Read the model definition and answer for the solid it produces. Units are mm, in the model's axes. Coordinates: 2 decimals unless noted, no trailing zeros. Write each loop counter-clockwise with the first axis right and the second up, starting at its lowest first coordinate (ties: lowest second). Pieces come first, ordered by that corner, then holes. Notation, with made-up numbers: (69.25, 49.25) -> (81.25, 49.25) arc R15 cw to (81.25, 56.25) -> close; hole circle Ø8 at (-0.75, 66.5). An arc over 180 degrees is marked (long way). Answer in a Markdown table with one row per item. Add a question column.
Item 1: For a pull along Z with two mould halves and no side action, classify faces 1 (the face through (-5, 4, -4)), 2 (the face through (-4.346, 1.972, -0.834)), 3 (the face through (5.854, 3.865, -14.543)) as +Z half, -Z half, draft (parallel to the pull), parting line (faces both ways), or undercut.
Item 2: Section A-A on z = -1.5 is taken. Write down the section's boundary in (x, y).
Item 3: Straight lines are drawn through the part: line 1 (X direction, y = 1.35, z = -0.5); line 2 (Z direction, x = 3, y = 3.55); line 3 (Z direction, x = 5.5, y = 2.65). For each, find the intervals that lie inside material, in ascending order. Write a range as from..to.
Item 4: Section B-B on y = 2.25 is taken. Write down the section's boundary in (x, z), then the cut area to 3 significant figures.
```python
from build123d import *

# Parameters (mm, degrees)
SKETCH1_W                      = 25
SKETCH1_H                      = 25
BOSS_EXTRUDE1_DEPTH            = 4
FILLET1_R                      = 4
F_1_7_1_7_DIAMETER_HOLE1_D     = 1.7
F_1_7_1_7_DIAMETER_HOLE1_DEPTH = 8.5
CHAMFER1_SIZE                  = 0.5


with BuildPart() as part:
    # Sketch1 → Boss-Extrude1 (new body)
    with BuildSketch(Plane(origin=(0, 0, 0), x_dir=(1, 0, 0), z_dir=(0, 1, 0))):
        with Locations((-5.188287333, 3.444371681)):
            Rectangle(SKETCH1_W, SKETCH1_H)
    extrude(amount=BOSS_EXTRUDE1_DEPTH)

    # Fillet1
    fillet1_edges = [part.edges().sort_by_distance(p)[0] for p in [
        (-17.688287333, 2, -15.944371681),
        (7.311712667, 2, -15.944371681),
        (7.311712667, 2, 9.055628319),
        (-17.688287333, 2, 9.055628319),
    ]]
    fillet(fillet1_edges, radius=FILLET1_R)

    # Ø1.7 (1.7) Diameter Hole1
    with Locations(Plane(origin=(-5.188287333, 4, -0.944371681), x_dir=(0, 0, 1), z_dir=(0, 1, 0))):
        with Locations((0, 0)):
            Hole(F_1_7_1_7_DIAMETER_HOLE1_D / 2, depth=F_1_7_1_7_DIAMETER_HOLE1_DEPTH)

    # Chamfer1
    chamfer1_edges = [part.edges().sort_by_distance(p)[0] for p in [
        (-17.688287333, 0, -3.444371681),
        (-17.688287333, 4, -3.444371681),
        (-5.188287333, 0, -15.944371681),
        (7.311712667, 0, -3.444371681),
        (-5.188287333, 0, 9.055628319),
        (-16.516714458, 0, 7.884055444),
        (6.140139792, 0, 7.884055444),
        (6.140139792, 0, -14.772798805),
        (-16.516714458, 0, -14.772798805),
        (-5.188287333, 4, -15.944371681),
        (-5.188287333, 4, 9.055628319),
        (7.311712667, 4, -3.444371681),
        (-16.516714458, 4, 7.884055444),
        (6.140139792, 4, 7.884055444),
        (6.140139792, 4, -14.772798805),
        (-16.516714458, 4, -14.772798805),
    ]]
    chamfer(chamfer1_edges, length=CHAMFER1_SIZE)


solid = part.part
```
Results below:
| question | item | result |
|---|---|---|
| 1 | face 1 | draft |
| 1 | face 2 | undercut |
| 1 | face 3 | -Z half |
| 2 | outline | (-17.69, 0.5) -> (-17.19, 0) -> (-5.83, 0) -> (-5.83, 4) -> (-17.19, 4) -> (-17.69, 3.5) -> close; (-4.55, 0) -> (6.81, 0) -> (7.31, 0.5) -> (7.31, 3.5) -> (6.81, 4) -> (-4.55, 4) -> close |
| 3 | line 1 | x = -17.69..-5.91, -4.46..7.31 |
| 3 | line 2 | z = -15.89..9.01 |
| 3 | line 3 | z = -15.29..8.4 |
| 4 | outline | (-17.69, -11.94) arc R4 ccw to (-13.69, -15.94) -> (3.31, -15.94) arc R4 ccw to (7.31, -11.94) -> (7.31, 5.06) arc R4 ccw to (3.31, 9.06) -> (-13.69, 9.06) arc R4 ccw to (-17.69, 5.06) -> close; hole circle Ø1.7 at (-5.19, -0.94) |
| 4 | area | 609 mm2 |
